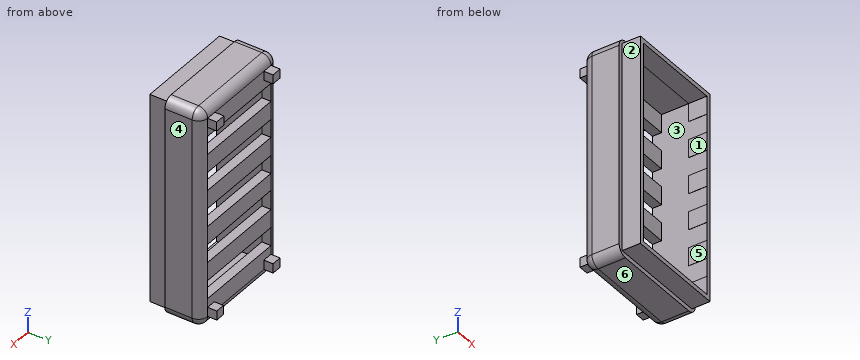
from build123d import *

# Parameters (mm, degrees)
F0_W      = 55
F0_H      = 115
F0_W_2    = 50
F0_H_2    = 110
F1_DEPTH  = 20
F3_W      = 55
F3_H      = 115
F5_DEPTH  = 10
F6_W      = 50
F6_H      = 110
F7_DEPTH  = 215.8
F8_W      = 60
F8_H      = 120
F9_DEPTH  = 5
F10_W     = 50
F10_H     = 10
F12_DEPTH = 30.001
F13_R     = 4.99999
F14_W     = 5.7372912765
F14_H     = 5
F14_W_2   = 5.2530970424
F14_H_2   = 5.0719603896
F15_DEPTH = 5
F16_W     = 5.5731512606
F16_H     = 5
F16_H_2   = 5.1789134741
F17_DEPTH = 5


# Not quite as in the source:
# - a fillet or chamfer is up to 0.001 mm smaller than in the source, because OpenCascade refuses the exact size


with BuildPart() as f1:
    # F0 (on Front) → F1 (new body)
    with BuildSketch(Plane.XZ):
        Polygon((-31.2259571254, 74.3091152272), (-33.7259571254, 74.3091152272), (-33.7259571254, -45.6908847728), (26.2740428746, -45.6908847728), (26.2740428746, 74.3091152272), align=None)
        with Locations((-3.7259571254, 14.3091152272)):
            Rectangle(F0_W, F0_H, mode=Mode.SUBTRACT)
        with Locations((-3.7259571254, 14.3091152272)):
            Rectangle(F0_W, F0_H)
        with Locations((-3.7259571254, 14.3091152272)):
            Rectangle(F0_W_2, F0_H_2, mode=Mode.SUBTRACT)
    extrude(amount=F1_DEPTH)

    # F3 (on offset) + F4 (on offset) → F5 (join)
    with BuildSketch(Plane.XZ.offset(20)):
        with Locations((-3.8123092055, 14.2757248878)):
            Rectangle(F3_W, F3_H)
    with BuildSketch(Plane.XZ.offset(20)):
        Polygon((-28.6821052432, -40.8934615552), (21.3168207556, -40.8934615552), (20.2441066504, 69.0581277013), (-28.6821052432, 69.0581277013), align=None)
    extrude(amount=F5_DEPTH)

    # F6 (on face) → F7 (cut)
    with BuildSketch(Plane.XZ.offset(30)):
        with Locations((-3.8123092055, 14.2757248878)):
            Rectangle(F6_W, F6_H)
    extrude(amount=-F7_DEPTH, mode=Mode.SUBTRACT)

    # F8 (on face) → F9 (join)
    with BuildSketch(Plane(origin=(0, 0, 0), x_dir=(-1, 0, 0), z_dir=(0, 1, 0))):
        with Locations((3.7259571254, 14.3091152272)):
            Rectangle(F8_W, F8_H)
    extrude(amount=-F9_DEPTH)

    # F10 (on face) → F12 (cut, through all)
    with BuildSketch(Plane(origin=(0, 0, 0), x_dir=(-1, 0, 0), z_dir=(0, 1, 0))):
        with Locations((3.7259571254, 54.3091152272)):
            Rectangle(F10_W, F10_H)
        with Locations((3.7259571254, 34.3091152272)):
            Rectangle(F10_W, F10_H)
        with Locations((3.7259571254, 14.3091152272)):
            Rectangle(F10_W, F10_H)
        Polygon((-21.2740428746, -0.6908847728), (-21.2740428746, -10.6908847728), (28.7259571254, -10.6908847728), (28.7259571254, 0), align=None)
        with Locations((3.7259571254, -25.6908847728)):
            Rectangle(F10_W, F10_H)
    extrude(amount=-F12_DEPTH, mode=Mode.SUBTRACT)

    # F13 (radius 5 in the source; OpenCascade refuses exactly that, so slightly less here)
    f13_edges = [f1.edges().sort_by_distance(p)[0] for p in [
        (-3.725957, 0, -45.690885),
        (-33.725957, 0, 14.309115),
        (26.274043, 0, 14.309115),
        (-3.725957, 0, 74.309115),
        (26.274043, -10, -45.690885),
        (26.274043, -10, 74.309115),
        (-33.725957, -10, -45.690885),
        (-33.725957, -10, 74.309115),
    ]]
    fillet(f13_edges, radius=F13_R)

    # F14 (on face) → F15 (join)
    with BuildSketch(Plane(origin=(0, 0, 0), x_dir=(-1, 0, 0), z_dir=(0, 1, 0))):
        with Locations((-18.4053972363, 66.8091152272)):
            Rectangle(F14_W, F14_H)
        with Locations((-18.5921611264, -38.1038859487)):
            Rectangle(F14_W_2, F14_H_2)
    extrude(amount=F15_DEPTH)

    # F16 (on face) → F17 (join)
    with BuildSketch(Plane(origin=(0, 0, 0), x_dir=(-1, 0, 0), z_dir=(0, 1, 0))):
        with Locations((25.9393814951, 66.8091152272)):
            Rectangle(F16_W, F16_H)
        with Locations((25.9393814951, -38.0802713335)):
            Rectangle(F16_W, F16_H_2)
    extrude(amount=F17_DEPTH)


solid = f1.part
Could you check a few things on this model? Use its own coordinates, in mm. Face numbers are marked on the shaded views. A direction names the side the tool comes from. Coordinates: 2 decimals unless noted, no trailing zeros. Write each loop counter-clockwise with the first axis right and the second up, starting at its lowest first coordinate (ties: lowest second). Pieces come first, ordered by that corner, then holes. Notation, with made-up numbers: (55.25, -33) - (91.25, -33) arc R23 cw to (91.25, -11) - close; hole circle Ø1 at (85, 43). An arc over 180 degrees is marked (long way). Put each result on its own line as item: value. Start each with the question number.
Q1. Which directions (+Z, -Z, +X, -X, +Y, -Y) give clear straight access to the entire face, cutting with the end or side of a thin tool? Please do the marked faces 1, 2 and 3.
Q2. I want a section at A-A on y = 2. Write out the boundary of the cut face in (x, z).
Q3. Please list where these lines run through material, in increasing order: L1, parallel to Z at x = 17, y = -16.5; L2, parallel to Z at x = -24.5, y = -26; L3, parallel to X at y = -22.5, z = 21.
Q4. I want a section at D-D on y = -3. Write out the boundary of the cut face in (x, z).
Q5. Thinking about a two-plate mould opening in Z: for the marked faces 4, 5 and 6, which applies, pulls with the +Z half, pulls with the -Z half, needs draft (parallel to the pull), parting line crosses it, or undercut?
Q6. I'm going to push flat-ended pins straight in: P1, Ø3, axis at x = -3, z = 62.5, coming from the +Y side; P2, Ø4, axis at y = 1.5, z = -39, coming from the -X side; P3, Ø12, axis at x = 0.5, z = -32, coming from the -Y side. Where does each tip first touch, or does it pass through?
Checks:
1. face 1: -Y
1. face 2: +Z, -Z, -X, -Y
1. face 3: none
2. outline: (-28.73, -40.67) - (-23.15, -40.67) - (-23.15, -35.49) - (-28.73, -35.49) - close; (-28.73, 64.31) - (-23.15, 64.31) - (-23.15, 69.31) - (-28.73, 69.31) - close; (15.54, 64.31) - (21.27, 64.31) - (21.27, 69.31) - (15.54, 69.31) - close; (15.97, -40.64) - (21.22, -40.64) - (21.22, -35.57) - (15.97, -35.57) - close
3. L1: -45.69 to -40.72, 69.31 to 74.31
3. L2: -43.22 to -40.72, 69.28 to 71.78
3. L3: -31.31 to -28.81, 21.19 to 23.69
4. outline: (-33.31, -40.69) arc R4.58 ccw to (-28.73, -45.27) - (21.27, -45.27) arc R4.58 ccw to (25.86, -40.69) - (25.86, 69.31) arc R4.58 ccw to (21.27, 73.89) - (-28.73, 73.89) arc R4.58 ccw to (-33.31, 69.31) - close; hole (-28.73, -30.69) - (21.27, -30.69) - (21.27, -20.69) - (-28.73, -20.69) - close; hole (-28.73, -10.69) - (21.27, -10.69) - (21.27, -0.69) - (-28.73, 0) - close; hole (-28.73, 9.31) - (21.27, 9.31) - (21.27, 19.31) - (-28.73, 19.31) - close; hole (-28.73, 29.31) - (21.27, 29.31) - (21.27, 39.31) - (-28.73, 39.31) - close; hole (-28.73, 49.31) - (21.27, 49.31) - (21.27, 59.31) - (-28.73, 59.31) - close
5. face 4: needs draft
5. face 5: undercut
5. face 6: pulls with the -Z half
6. P1: y = 0
6. P2: x = -30.91
6. P3: y = -5
